from build123d import *

# Parameters (mm, degrees)
F0_W      = 212
F0_H      = 72
F1_DEPTH  = 5.5
F2_R      = 15
F3_W      = 45.625
F3_H      = 5.5
F4_DEPTH  = 12
F6_DEPTH  = 2
F7_R      = 10.5
F8_R      = 11.5
F9_R      = 14
F10_R     = 15
F11_W     = 153
F11_H     = 55
F12_DEPTH = 4
F14_D     = 3.4


# Not quite as in the source:
# - a feature names something its author has since deleted; it is built from what else it names


with BuildPart() as f1:
    # F0 (on Top) → F1 (new body)
    with BuildSketch(Plane.XY):
        Rectangle(F0_W, F0_H)
    extrude(amount=F1_DEPTH)

    # F2
    f2_edges = [f1.edges().sort_by_distance(p)[0] for p in [
        (-106, -36, 2.75),
        (106, -36, 2.75),
    ]]
    fillet(f2_edges, radius=F2_R)

    # F3 (on face) → F4 (cut)
    with BuildSketch(Plane.XZ.offset(36)):
        with Locations((-53.6875, 2.75)):
            Rectangle(F3_W, F3_H)
        with Locations((53.6875, 2.75)):
            Rectangle(F3_W, F3_H)
    extrude(amount=-F4_DEPTH, mode=Mode.SUBTRACT)

    # F5 (on face) → F6 (join)
    with BuildSketch(Plane(origin=(0, 0, 0), x_dir=(1, 0, 0), z_dir=(0, 0, -1))):
        Polygon((-105, -7.5), (-106, -7.5), (-106, -36), (106, -36), (106, -7.5), (105, -7.5), (105, -35), (-105, -35), align=None)
        Polygon((101.5, -31.5), (-101.5, -31.5), (-101.5, -7.5), (-102.5, -7.5), (-102.5, -32.5), (102.5, -32.5), (102.5, -7.5), (101.5, -7.5), align=None)
    extrude(amount=F6_DEPTH)

    # F7
    f7_edges = [f1.edges().sort_by_distance(p)[0] for p in [
        (101.5, 31.5, -1),
        (-101.5, 31.5, -1),
    ]]
    fillet(f7_edges, radius=F7_R)

    # F8
    f8_edges = [f1.edges().sort_by_distance(p)[0] for p in [
        (102.5, 32.5, -1),
        (-102.5, 32.5, -1),
    ]]
    fillet(f8_edges, radius=F8_R)

    # F9
    f9_edges = [f1.edges().sort_by_distance(p)[0] for p in [
        (105, 35, -1),
        (-105, 35, -1),
    ]]
    fillet(f9_edges, radius=F9_R)

    # F10
    f10_edges = [f1.edges().sort_by_distance(p)[0] for p in [
        (106, 36, 1.75),
        (-106, 36, 1.75),
    ]]
    fillet(f10_edges, radius=F10_R)

    # F11 (on face) → F12 (cut)
    with BuildSketch(Plane.XY.offset(5.5)):
        with Locations((0, 6)):
            Rectangle(F11_W, F11_H)
    extrude(amount=-F12_DEPTH, mode=Mode.SUBTRACT)

    # F14 (through all)
    with Locations(Plane.XY.offset(5.5)):
        with Locations((-85.5, 15.5), (85.5, 15.5), (85.5, -15.5), (-85.5, -15.5)):
            Hole(F14_D / 2)


solid = f1.part
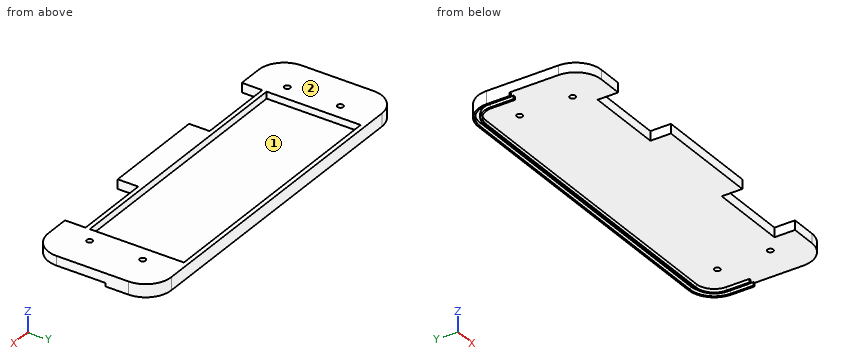
The model under review builds one solid part; all positions refer to its coordinate system, in mm. Face numbers are marked on the shaded views. Round coordinates to 2 decimals unless told otherwise and drop trailing zeros. Order: outer loops, then holes, each group sorted by start corner. A loop starts at its lowest first (then second) coordinate and runs counter-clockwise, first axis right, second up. Notation, with made-up numbers: (-23.75, 75) -> (-10.75, 75) arc R10 ccw to (-10.75, 92) -> close; hole circle Ø2 at (88, 1.5). An arc over 180 degrees is marked (long way). Write item = value, one per line. Start each with the question number.
Item 1: Consider section A-A on z = 3.5. Write out the cut boundary in (x, y) (3 decimals), plus the area to 3 significant figures.
Item 2: Clearance check with flat-ended pins moving along their axes: pin 1 Ø3 at (x, z) = (-53.5, 1.5) entering from -Y; pin 2 Ø21.5 at (x, y) = (46, -9) entering from -Z; pin 3 Ø1 at (x, z) = (-10.5, -1) entering from -Y. State where each tip first meets the part, or that it passes through.
Item 3: For line 1 along Y through (x, z) = (85.5, 3.85); line 2 along X through (y, z) = (14, -0.75); line 3 along Y through (x, z) = (36.5, -0.5), list the stretches that pass through material, from the lowest coordinate up.
Item 4: Consider section D-D on x = -1. Write out the cut boundary in (y, z), plus the area to 3 significant figures.
Item 5: Mouldability with a two-part tool opening along X and no side actions: class the marked faces 1 and 2 as released by +X, released by -X, zero draft, split by the parting line, or undercut.
Item 6: Consider section C-C on y = 10.5. Write out the cut boundary in (x, z), plus the area to 3 significant figures.
Item 7: Consider section B-B on x = 42.5. Write out the cut boundary in (y, z).
Conclusion:
q1.outline = (-106, -21) arc R15 ccw to (-91, -36) -> (-76.5, -36) -> (-76.5, -24) -> (-30.875, -24) -> (-30.875, -36) -> (30.875, -36) -> (30.875, -24) -> (76.5, -24) -> (76.5, -36) -> (91, -36) arc R15 ccw to (106, -21) -> (106, 21) arc R15 ccw to (91, 36) -> (-91, 36) arc R15 ccw to (-106, 21) -> close; hole circle Ø3.4 at (-85.5, -15.5); hole circle Ø3.4 at (-85.5, 15.5); hole (-76.5, -21.5) -> (76.5, -21.5) -> (76.5, 33.5) -> (-76.5, 33.5) -> close; hole circle Ø3.4 at (85.5, -15.5); hole circle Ø3.4 at (85.5, 15.5)
q1.area = 5,520 mm2
q2.pin_1 = -24
q2.pin_2 = 0
q2.pin_3 = 31.5
q3.line_1 = -36 to -17.2, -13.8 to 13.8, 17.2 to 36
q3.line_2 = -106 to -105, -102.5 to -101.5, 101.5 to 102.5, 105 to 106
q3.line_3 = 31.5 to 32.5, 35 to 36
q4.outline = (-36, 0) -> (31.5, 0) -> (31.5, -2) -> (32.5, -2) -> (32.5, 0) -> (35, 0) -> (35, -2) -> (36, -2) -> (36, 5.5) -> (33.5, 5.5) -> (33.5, 1.5) -> (-21.5, 1.5) -> (-21.5, 5.5) -> (-36, 5.5) -> close
q4.area = 180 mm2
q5.face_1 = undercut
q5.face_2 = zero draft
q6.outline = (-106, -2) -> (-105, -2) -> (-105, 0) -> (-102.5, 0) -> (-102.5, -2) -> (-101.5, -2) -> (-101.5, 0) -> (101.5, 0) -> (101.5, -2) -> (102.5, -2) -> (102.5, 0) -> (105, 0) -> (105, -2) -> (106, -2) -> (106, 5.5) -> (76.5, 5.5) -> (76.5, 1.5) -> (-76.5, 1.5) -> (-76.5, 5.5) -> (-106, 5.5) -> close
q6.area = 562 mm2
q7.outline = (-24, 0) -> (31.5, 0) -> (31.5, -2) -> (32.5, -2) -> (32.5, 0) -> (35, 0) -> (35, -2) -> (36, -2) -> (36, 5.5) -> (33.5, 5.5) -> (33.5, 1.5) -> (-21.5, 1.5) -> (-21.5, 5.5) -> (-24, 5.5) -> close
